Could you check a few things on this model? Use its own coordinates, in mm. Face numbers are marked on the shaded views. A direction names the side the tool comes from. Give positions to 0.01 mm unless a question says otherwise; leave off trailing zeros. Order: outer loops, then holes, each group sorted by start corner. A loop starts at its lowest first (then second) coordinate and runs counter-clockwise, first axis right, second up. Notation, with made-up numbers: (6, -27) -> (34, -27) arc R22 cw to (34, -5) -> close; hole circle Ø6 at (31, 21). An arc over 180 degrees is marked (long way). One line per item, written item: value.
```python
from build123d import *

# Parameters (mm, degrees)
BOSS_EXTRU_1_DEPTH      = 39
ESQUISSE2_R             = 1.25
ENL_V_MAT_EXTRU_1_DEPTH = 39
ESQUISSE3_R             = 11
ESQUISSE3_R_2           = 4.6
BOSS_EXTRU_2_DEPTH      = 2
ESQUISSE4_R             = 2.5
BOSS_EXTRU_3_DEPTH      = 22.5
ENL_V_START             = -7
ENL_V_MAT_EXTRU_4_DEPTH = 7
ESQUISSE9_W             = 16
ESQUISSE9_H             = 10
BOSS_EXTRU_4_DEPTH      = 6.3


with BuildPart() as part:
    # Esquisse1 → Boss.-Extru.1 (new body)
    with BuildSketch(Plane(origin=(0, 0, 0), x_dir=(1, 0, 0), z_dir=(0, 1, 0))):
        Polygon((3.535533906, 2.549558154), (0, 6.08509206), (0, 41.014024248), (3.535533906, 44.549558154), (38.464466094, 44.549558154), (42, 41.014024248), (42, 6.08509206), (38.464466094, 2.549558154), align=None)
    extrude(amount=BOSS_EXTRU_1_DEPTH)

    # Esquisse2 → Enlèv. mat.-Extru.1 (cut)
    with BuildSketch(Plane(origin=(0, 39, 0), x_dir=(1, 0, 0), z_dir=(0, 1, 0))):
        with Locations(Location((5.3, 39.249558154, 0), (0, 0, 270))):
            Circle(ESQUISSE2_R)
        with Locations(Location((36.7, 39.249558154, 0), (0, 0, 270))):
            Circle(ESQUISSE2_R)
        with Locations(Location((36.7, 7.849558154, 0), (0, 0, 270))):
            Circle(ESQUISSE2_R)
        with Locations(Location((5.3, 7.849558154, 0), (0, 0, 270))):
            Circle(ESQUISSE2_R)
    extrude(amount=-ENL_V_MAT_EXTRU_1_DEPTH, mode=Mode.SUBTRACT)

    # Esquisse3 → Boss.-Extru.2 (add)
    with BuildSketch(Plane(origin=(0, 39, 0), x_dir=(1, 0, 0), z_dir=(0, 1, 0))):
        with Locations(Location((21, 23.549558154, 0), (0, 0, 90))):
            Circle(ESQUISSE3_R)
        with Locations(Location((21, 23.549558154, 0), (0, 0, 270))):
            Circle(ESQUISSE3_R_2, mode=Mode.SUBTRACT)
    extrude(amount=BOSS_EXTRU_2_DEPTH)

    # Esquisse4 → Boss.-Extru.3 (add)
    with BuildSketch(Plane(origin=(0, 39, 0), x_dir=(1, 0, 0), z_dir=(0, 1, 0))):
        with Locations(Location((21, 23.549558154, 0), (0, 0, 90))):
            Circle(ESQUISSE4_R)
    extrude(amount=BOSS_EXTRU_3_DEPTH)

    # Esquisse8 → Enlèv. mat.-Extru.4 (cut)
    with BuildSketch(Plane(origin=(0, 61.5, 0), x_dir=(1, 0, 0), z_dir=(0, 1, 0)).offset(ENL_V_START)):
        with BuildLine():
            Line((22.47490916, 21.530983664), (19.52509084, 21.530983664))
            ThreePointArc((19.52509084, 21.530983664), (21, 21.049558154), (22.47490916, 21.530983664))
        make_face()
    extrude(amount=ENL_V_MAT_EXTRU_4_DEPTH, mode=Mode.SUBTRACT)

    # Esquisse9 → Boss.-Extru.4 (add)
    with BuildSketch(Plane(origin=(42, 0, 0), x_dir=(0, 0, -1), z_dir=(1, 0, 0))):
        with Locations((23.549024248, 5)):
            Rectangle(ESQUISSE9_W, ESQUISSE9_H)
    extrude(amount=BOSS_EXTRU_4_DEPTH)


solid = part.part
```
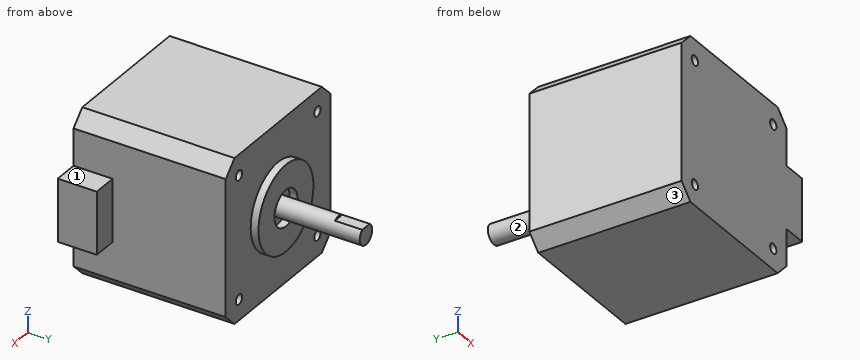
1) Suppose I cut it at B-B, the plane y = 40. Write out the boundary of the cut face in (x, z).
Answer below:
outline: circle Ø22 at (21, -23.55); circle Ø5 at (21, -23.55); hole circle Ø9.2 at (21, -23.55)
2) Suppose I cut it at C-C, the plane z = -8. Write out the boundary of the cut face in (x, y).
Answer below:
outline: (0, 0) -> (4.06, 0) -> (4.06, 39) -> (0, 39) -> close; (6.54, 0) -> (35.46, 0) -> (35.46, 39) -> (6.54, 39) -> close; (37.94, 0) -> (42, 0) -> (42, 39) -> (37.94, 39) -> close
3) Suppose I cut it at A-A, the plane x = 5.3. Write out the boundary of the cut face in (y, z), then the cut area to 3 significant figures.
Answer below:
outline: (0, -44.55) -> (39, -44.55) -> (39, -40.5) -> (0, -40.5) -> close; (0, -38) -> (39, -38) -> (39, -9.1) -> (0, -9.1) -> close; (0, -6.6) -> (39, -6.6) -> (39, -2.55) -> (0, -2.55) -> close
area: 1,440 mm2
4) For P1, Ø5, axis at x = 44, z = -26.5, coming from the +Y side; P2, Ø3, axis at x = 15.5, y = 42, coming from the +Z side; P3, Ø3, axis at x = 44, y = 5, coming from the +Z side; P4, Ø2, axis at x = 36.7, z = -7.85, coming from the +Y side (1 decimal), each with a flat end and sliding along its axis, tell me the tip position at first contact or that it passes through.
Answer below:
P1: stops at y = 39
P2: stops at z = -13.46
P3: stops at z = -15.55
P4: passes through
5) If I drill on line 1 along Z through (x, y) = (36, 9); line 2 along X through (y, z) = (16.5, -38.5); line 3 along Y through (x, z) = (11, -7), over which ranges is the centre line in solid material (lowest first)?
Answer below:
line 1: z = -44.55 to -40.29, -38.21 to -8.89, -6.81 to -2.55
line 2: x = 0 to 4.3, 6.3 to 35.7, 37.7 to 42
line 3: y = 0 to 39
6) For the marked faces 1, 2 and 3, which set-ups out of +Z, -Z, +X, -X, +Y, -Y let a thin tool reach every point of the face, with its end or its side?
Answer below:
face 1: +Z, +X, +Y, -Y
face 2: +Y
face 3: -Z, -X, +Y, -Y
7) Suppose I cut it at D-D, the plane x = 21. Write out the boundary of the cut face in (y, z).
Answer below:
outline: (0, -44.55) -> (39, -44.55) -> (39, -34.55) -> (41, -34.55) -> (41, -28.15) -> (39, -28.15) -> (39, -26.05) -> (61.5, -26.05) -> (61.5, -21.53) -> (54.5, -21.53) -> (54.5, -21.05) -> (39, -21.05) -> (39, -18.95) -> (41, -18.95) -> (41, -12.55) -> (39, -12.55) -> (39, -2.55) -> (0, -2.55) -> close
